Read the model definition and answer for the solid it produces. Units are mm, in the model's axes. A direction names the side the tool comes from. Coordinates: 2 decimals unless noted, no trailing zeros. Order: outer loops, then holes, each group sorted by start corner. A loop starts at its lowest first (then second) coordinate and runs counter-clockwise, first axis right, second up. Notation, with made-up numbers: (68, 83) - (108, 83) arc R24 ccw to (108, 99) - close; hole circle Ø3 at (-7, 80). An arc over 180 degrees is marked (long way). Answer as a JSON object with one key per item and string values. Group by question number.
from build123d import *

# Parameters (mm, degrees)
F0_W      = 72
F0_H      = 132
F1_DEPTH  = 17.7
F2_W      = 66
F2_H      = 126
F3_DEPTH  = 14.7
F4_W      = 72
F4_H      = 132
F4_W_2    = 66
F4_H_2    = 126
F4_W_3    = 63
F4_H_3    = 123
F5_DEPTH  = 1.2
F6_R      = 7.5
F7_DEPTH  = 25
F8_DEPTH  = 25
F9_R      = 5
F10_DEPTH = 25
F11_W     = 14
F11_H     = 6.5
F12_DEPTH = 25
F13_W     = 35
F13_H     = 3
F14_DEPTH = 25
F15_W     = 6.5
F15_H     = 45
F16_DEPTH = 25
F17_R     = 5
F18_DEPTH = 25
F19_R     = 7
F20_W     = 10.5434343904
F20_H     = 1.1330954731
F20_W_2   = 10.2601605222
F20_H_2   = 0.8498206735
F20_H_3   = 1.1330917478
F21_DEPTH = 81


with BuildPart() as f1:
    # F0 (on Front) → F1 (new body)
    with BuildSketch(Plane.XZ):
        Rectangle(F0_W, F0_H)
    extrude(amount=F1_DEPTH)

    # F2 (on face) → F3 (cut, through all)
    with BuildSketch(Plane.XZ.offset(17.7)):
        Rectangle(F2_W, F2_H)
    extrude(amount=-F3_DEPTH, mode=Mode.SUBTRACT)

    # F4 (on face) → F5 (join)
    with BuildSketch(Plane.XZ.offset(17.7)):
        Rectangle(F4_W, F4_H)
        Rectangle(F4_W_2, F4_H_2, mode=Mode.SUBTRACT)
        Rectangle(F4_W_2, F4_H_2)
        Rectangle(F4_W_3, F4_H_3, mode=Mode.SUBTRACT)
    extrude(amount=F5_DEPTH)

    # F6 (on face) → F7 (cut)
    with BuildSketch(Plane.XZ.offset(3)):
        with Locations((0, 50)):
            Circle(F6_R)
    extrude(amount=-F7_DEPTH, mode=Mode.SUBTRACT)

    # F6 (on face) → F8 (cut)
    with BuildSketch(Plane.XZ.offset(3)):
        with Locations((0, 50)):
            Circle(F6_R)
    extrude(amount=-F8_DEPTH, mode=Mode.SUBTRACT)

    # F9 (on face) → F10 (cut)
    with BuildSketch(Plane.XZ.offset(3)):
        with Locations((0, 39.799913764)):
            Circle(F9_R)
    extrude(amount=-F10_DEPTH, mode=Mode.SUBTRACT)

    # F11 (on face) → F12 (cut)
    with BuildSketch(Plane.XY.offset(66)):
        with Locations((0, -12.15)):
            Rectangle(F11_W, F11_H)
    extrude(amount=-F12_DEPTH, mode=Mode.SUBTRACT)

    # F13 (on face) → F14 (cut)
    with BuildSketch(Plane.XZ.offset(3)):
        with Locations((0, -54)):
            Rectangle(F13_W, F13_H)
    extrude(amount=-F14_DEPTH, mode=Mode.SUBTRACT)

    # F15 (on face) → F16 (cut)
    with BuildSketch(Plane.YZ.offset(36)):
        with Locations((-15.65, 28.5)):
            Rectangle(F15_W, F15_H)
    extrude(amount=-F16_DEPTH, mode=Mode.SUBTRACT)

    # F17 (on face) → F18 (cut)
    with BuildSketch(Plane.XY.offset(66)):
        with Locations((21.231278264, -7.4096710059)):
            Circle(F17_R)
    extrude(amount=-F18_DEPTH, mode=Mode.SUBTRACT)

    # F19
    f19_edges = [f1.edges().sort_by_distance(p)[0] for p in [
        (-36, -9.45, 66),
        (36, -9.45, 66),
        (-36, -9.45, -66),
        (36, -9.45, -66),
    ]]
    fillet(f19_edges, radius=F19_R)

    # F20 (on face) → F21 (cut)
    with BuildSketch(Plane(origin=(-36, 0, 0), x_dir=(0, -1, 0), z_dir=(-1, 0, 0))):
        with Locations((13.6282828048, 39.2333660275)):
            Rectangle(F20_W, F20_H)
        with Locations((13.7699197389, 6.2320143916)):
            Rectangle(F20_W_2, F20_H_2)
        with Locations((13.7699197389, -34.4177186489)):
            Rectangle(F20_W_2, F20_H_3)
    extrude(amount=-F21_DEPTH, mode=Mode.SUBTRACT)


solid = f1.part
1. A cutting plane is placed at B-B on x = 0. Write down the section's boundary in (y, z), and give its area (3 significant figures).
2. Straight lines are drawn through the part: L1, parallel to Z at x = 0, y = -1; L2, parallel to X at y = -2.1, z = 50; L3, parallel to X at y = -17.25, z = -42.5. For each, find the intervals that lie inside material, in ascending order.
3. A cutting plane is placed at A-A on x = -14. Write down the section's boundary in (y, z), and give its area (3 significant figures).
4. For faces 4 (the flat face through (0, -10, -63)), 5 (the flat face through (0, -8.9, 65)), 6 (the flat face through (34, -10, 6.657)), determine the directions among +Z, -Z, +X, -X, +Y, -Y from which every point of the face is accessible in a straight line to the end or side of a thin tool.
5. Given pin 1 (5 mm diameter, centred on x = -33.5, y = -13.5, fed in from +Z); pin 2 (5 mm diameter, centred on x = -34, y = -16, fed in from -Z); pin 3 (10 mm diameter, centred on x = -21.5, z = -37.5, fed in from -Y), each flat-ended and moving along its own axis, determine where each tip first touches the part or whether it passes through.
6. For a pull along Y with two mould halves and no side action, classify faces 1 (the flat face through (35, -12.4, 45)), 2 (the flat face through (0, -9, -66)), 3 (the flat face through (33, -10, -1)) as pulls with the +Y half, pulls with the -Y half, needs draft (parallel to the pull), parting line crosses it, or undercut.
7. A cutting plane is placed at C-C on z = -27.5. Write down the section's boundary in (x, y), and give its area (3 significant figures).
8. A cutting plane is placed at D-D on y = -10.75. State how many separate pieces and enclosed holes the cut face has, and give its area (3 significant figures).
Derived:
{
 "1": {"outline": "(-18.9, -66) - (0, -66) - (0, -55.5) - (-3, -55.5) - (-3, -63) - (-17.7, -63) - (-17.7, -61.5) - (-18.9, -61.5) - close; (-18.9, 61.5) - (-17.7, 61.5) - (-17.7, 63) - (-15.4, 63) - (-15.4, 66) - (-18.9, 66) - close; (-8.9, 63) - (-3, 63) - (-3, 57.5) - (0, 57.5) - (0, 66) - (-8.9, 66) - close; (-3, -52.5) - (0, -52.5) - (0, 34.8) - (-3, 34.8) - close", "area": "398 mm2"},
 "2": {"L1": "z = -66 to -55.5, -52.5 to 34.8, 57.5 to 66", "L2": "x = -36 to -7.5, 7.5 to 36", "L3": "x = -36 to -33, 33 to 36"},
 "3": {"outline": "(-18.9, -66) - (0, -66) - (0, -55.5) - (-3, -55.5) - (-3, -63) - (-17.7, -63) - (-17.7, -61.5) - (-18.9, -61.5) - close; (-18.9, 61.5) - (-17.7, 61.5) - (-17.7, 63) - (-3, 63) - (-3, -52.5) - (0, -52.5) - (0, 66) - (-18.9, 66) - close", "area": "486 mm2"},
 "4": {"face 4": "none", "face 5": "+Z", "face 6": "+X, -X, -Y"},
 "5": {"pin 1": "stops at z = 65.71", "pin 2": "stops at z = -65.54", "pin 3": "stops at y = -3"},
 "6": {"face 1": "pulls with the -Y half", "face 2": "needs draft", "face 3": "undercut"},
 "7": {"outline": "(-36, -18.9) - (-31.5, -18.9) - (-31.5, -17.7) - (-33, -17.7) - (-33, -3) - (33, -3) - (33, -17.7) - (31.5, -17.7) - (31.5, -18.9) - (36, -18.9) - (36, 0) - (-36, 0) - close", "area": "315 mm2"},
 "8": {"separate pieces": "8", "enclosed holes": "0", "area": "1,060 mm2"}
}
